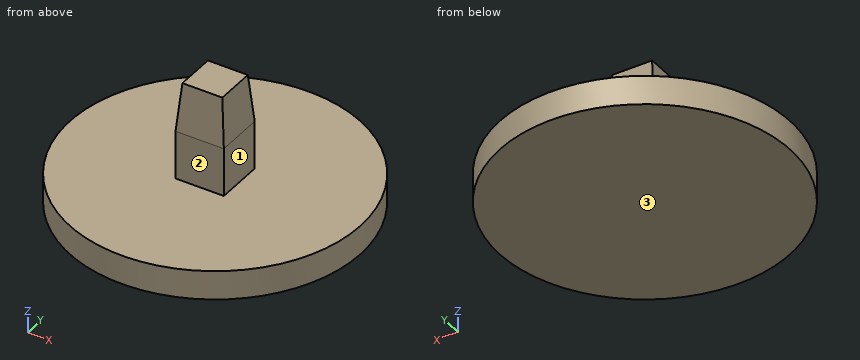
from build123d import *

# Parameters (mm, degrees)
F0_R      = 15
F0_W      = 5
F0_H      = 5
F1_DEPTH  = 3
F2_DEPTH  = 8
F2_FACE_W = 5
F2_FACE_H = 5
F3_DEPTH  = 5
F3_TAPER  = 5


with BuildPart() as f1:
    # F0 (on Top) → F1 (new body)
    with BuildSketch(Plane.XY):
        Circle(F0_R)
        Rectangle(F0_W, F0_H, mode=Mode.SUBTRACT)
    extrude(amount=F1_DEPTH)

    # F0 (on Top) → F2 (join)
    with BuildSketch(Plane.XY):
        Rectangle(F0_W, F0_H)
    extrude(amount=F2_DEPTH)

    # F2_face (on face) → F3 (join)
    with BuildSketch(Plane.XY.offset(8)):
        Rectangle(F2_FACE_W, F2_FACE_H)
    extrude(amount=F3_DEPTH, taper=F3_TAPER)


solid = f1.part
Check sheet for the modelled part. Datum: model origin and axes. Units: mm. Face numbers are marked on the shaded views. A direction names the side the tool comes from. Round coordinates to 2 decimals unless told otherwise and drop trailing zeros. Loops run counter-clockwise (first coordinate to the right, second up) from the corner with the lowest first, then second, coordinate; pieces in that order, holes last. Notation, with made-up numbers: M -15.5,-27 L 7.5,-27 A29 ccw 7.5,10 Z; hole C 3.25,31.5 d9. An arc over 180 degrees is marked long. One line per question, with ' | ' between items. Start each with the question number.
Item 1: Gauge pin test, flat ends, axial feed: pin 1 Ø1 at (y, z) = (-0.5, 10.5) entering from -X (3 decimals); pin 2 Ø5 at (y, z) = (3.5, 7) entering from +X; pin 3 Ø1.5 at (x, z) = (-1, 5) entering from -Y. Record the tip position at first contact, or that the pin passes through.
Item 2: Set-up check for the marked faces 1, 2 and 3: record each of +Z, -Z, +X, -X, +Y, -Y from which the full face is reachable in a straight line by a thin tool's end or side.
Item 3: Section check A-A (x = 0). Record the boundary of the cut face in (y, z).
Item 4: Section check C-C (z = 4.25). Record the boundary of the cut face in (x, y), and give its area (3 significant figures).
Item 5: Section check D-D (x = -8.25). Record the boundary of the cut face in (y, z).
Item 6: Scan lines: probe 1 along Z at (x, y) = (-3, 7); probe 2 along X at (y, z) = (0, 6.5); probe 3 along Y at (x, z) = (0, 1.75). Record each from-to range of solid material in increasing order.
Worked out:
1) pin 1: x = -2.325 | pin 2: x = 2.5 | pin 3: y = -2.5
2) face 1: +Z, +X, +Y, -Y | face 2: +Z, +X, -X, -Y | face 3: -Z, +X, -X, +Y, -Y
3) outline: M -15,0 L 15,0 L 15,3 L 2.5,3 L 2.5,8 L 2.06,13 L -2.06,13 L -2.5,8 L -2.5,3 L -15,3 Z
4) outline: M -2.5,-2.5 L 2.5,-2.5 L 2.5,2.5 L -2.5,2.5 Z | area: 25.0 mm^2
5) outline: M -12.53,0 L 12.53,0 L 12.53,3 L -12.53,3 Z
6) probe 1: 0 to 3 | probe 2: -2.5 to 2.5 | probe 3: -15 to 15
